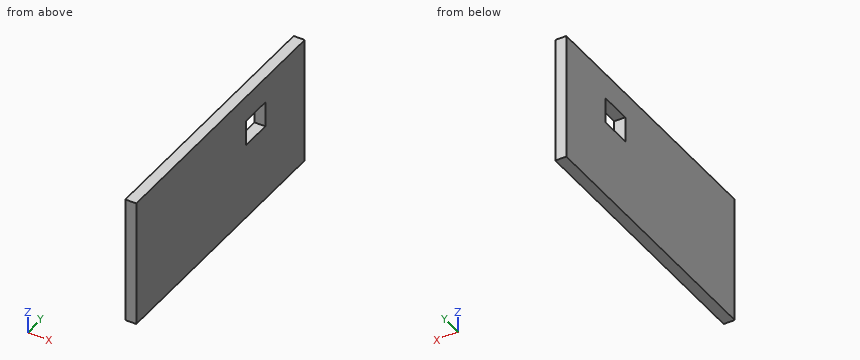
from build123d import *

# Parameters (mm, degrees)
SKETCH1_W           = 55
SKETCH1_H           = 120
BOSS_EXTRUDE1_DEPTH = 4.7625
SKETCH2_W           = 11
SKETCH2_H           = 14
CUT_EXTRUDE1_DEPTH  = 5.7625


with BuildPart() as part:
    # Sketch1 → Boss-Extrude1 (new body)
    with BuildSketch(Plane(origin=(0, 0, 0), x_dir=(0, 0, -1), z_dir=(1, 0, 0))):
        Rectangle(SKETCH1_W, SKETCH1_H)
    extrude(amount=BOSS_EXTRUDE1_DEPTH)

    # Sketch2 → Cut-Extrude1 (cut, through all)
    with BuildSketch(Plane.ZY):
        with Locations((11, 25)):
            Rectangle(SKETCH2_W, SKETCH2_H)
    extrude(amount=-CUT_EXTRUDE1_DEPTH, mode=Mode.SUBTRACT)


solid = part.part
Can you work these out from the model? Positions are in its coordinate system, mm. Coordinates: 2 decimals unless noted, no trailing zeros. Write each loop counter-clockwise with the first axis right and the second up, starting at its lowest first coordinate (ties: lowest second). Pieces come first, ordered by that corner, then holes. Notation, with made-up numbers: (-4.75, -27) -> (6.25, -27) arc R27 ccw to (6.25, -11) -> close; hole circle Ø3 at (-21.5, 60.5). An arc over 180 degrees is marked (long way). Write each question's results on one line, items separated by ' | '. Start each with the question number.
Q1. Imagine slicing it at B-B (x = 2.15). Write out the boundary of the cut face in (y, z).
Q2. Imagine slicing it at A-A (z = 9). Write out the boundary of the cut face in (x, y), then the cut area to 3 significant figures.
Q3. If I drill on probe 1 along Y at (x, z) = (4.3, 6), over which ranges is the centre line in solid material (lowest first)?
Q4. I'm going to push flat-ended pins straight in: pin 1 (8 mm diameter, centred on y = 26.5, z = 11.5, fed in from +X); pin 2 (4 mm diameter, centred on y = -3.5, z = 9, fed in from -X). Where does each tip first touch, or does it pass through?
Taken from the geometry:
1) outline: (-60, -27.5) -> (60, -27.5) -> (60, 27.5) -> (-60, 27.5) -> close; hole (18, 5.5) -> (32, 5.5) -> (32, 16.5) -> (18, 16.5) -> close
2) outline: (0, -60) -> (4.76, -60) -> (4.76, 18) -> (0, 18) -> close; (0, 32) -> (4.76, 32) -> (4.76, 60) -> (0, 60) -> close | area: 505 mm^2
3) probe 1: y = -60 to 18, 32 to 60
4) pin 1: passes through | pin 2: stops at x = 0
